Check sheet for the modelled part. Datum: model origin and axes. Units: mm. A direction names the side the tool comes from. Round coordinates to 2 decimals unless told otherwise and drop trailing zeros. Order: outer loops, then holes, each group sorted by start corner. A loop starts at its lowest first (then second) coordinate and runs counter-clockwise, first axis right, second up. Notation, with made-up numbers: (-13, 34.5) -> (29, 34.5) arc R32 cw to (29, 73.5) -> close; hole circle Ø1 at (48, 55.25). An arc over 180 degrees is marked (long way). Answer in a Markdown table with one row per item. Add a question column.
1. Material ranges on L1, parallel to Y at x = 5.25, z = 0; L2, parallel to Z at x = -0.25, y = 30.5; L3, parallel to Z at x = -4.5, y = 17.5, recorded low to high. Write a range as from..to.
2. Draft check along Z on faces 6 (the cylindrical face through (-3.51, 7.67, 4.23)), 7 (the cylindrical face through (2.6, 28.5, -0.3)), 8 (the cylindrical face through (4.904, 36.575, 0.129)). Enter one of: +Z half, -Z half, draft (parallel to the pull), parting line (faces both ways), or undercut.
3. Sectioned sample at A-A, the plane x = -3.25. Count the separate pieces of the cut face and the enclosed holes in it, then the cut area to 3 significant figures.
4. Sectioned sample at C-C, the plane z = 0. Record the boundary of the cut face in (x, y).
5. Sectioned sample at B-B, the plane z = 7.75. Record the boundary of the cut face in (x, y).
6. Depth check by flat-ended pin: P1, Ø3.5, axis at x = 2.48, y = 30.7, coming from the -Z side; P2, Ø5, axis at x = -2, y = 23.5, coming from the +Z side; P3, Ø0.6, axis at x = 3.5, y = 8, coming from the -Z side. Enter the tip coordinate at first touch or a pass-through.
7. Access from +Z, -Z, +X, -X, +Y, -Y to the whole of each face (thin tool, end or side, straight path). Record for faces 1 (the flat face through (4, 8, 5.334)), 2 (the flat face through (4, 8, -5.334)), 3 (the flat face through (-4, 17.653, 7)), 4 (the flat face through (0, 27, -5.88)), 5 (the cylindrical face through (-3.509, 7.669, -3.986)).
```python
from build123d import *

# Parameters (mm, degrees)
SKETCH1_R           = 1.905
SKETCH1_R_2         = 2.2178391
BOSS_EXTRUDE1_DEPTH = 7.76605
SKETCH2_W           = 9.0297
SKETCH2_H           = 6.858
CUT_EXTRUDE1_DEPTH  = 7.76605
CUT_EXTRUDE2_DEPTH  = 9.0297
SKETCH5_R           = 1.5875
CUT_EXTRUDE3_DEPTH  = 12.7
FILLET2_R           = 1.27
SKETCH6_W           = 4.445
SKETCH6_H           = 8.89
CUT_EXTRUDE4_DEPTH  = 8.636
SKETCH6_4_W         = 1.04775
SKETCH6_4_H         = 1.905
BOSS_EXTRUDE2_DEPTH = 15.5321
SKETCH7_R           = 2.661534018
CUT_EXTRUDE5_DEPTH  = 12.7
CUT_EXTRUDE6_DEPTH  = 8.636
CUT_EXTRUDE7_DEPTH  = 0.635
CUT_EXTRUDE8_DEPTH  = 0.635
SKETCH11_R          = 1.27
CUT_EXTRUDE9_DEPTH  = 12.7


with BuildPart() as part:
    # Sketch1 → Boss-Extrude1 (new, symmetric)
    with BuildSketch(Plane(origin=(0, 0, 0), x_dir=(0, 0, -1), z_dir=(1, 0, 0))):
        with BuildLine():
            Line((-9.779, 8.763), (-9.779, 21.463))
            Line((-9.779, 21.463), (-5.8801, 21.971))
            Line((-5.8801, 21.971), (-5.8801, 30.6959))
            ThreePointArc((-5.8801, 30.6959), (0, 36.576), (5.8801, 30.6959))
            Line((5.8801, 30.6959), (5.8801, 21.971))
            Line((5.8801, 21.971), (9.779, 21.463))
            Line((9.779, 21.463), (9.779, 8.763))
            Line((9.779, 8.763), (4.28625, 8.763))
            Line((4.28625, 8.763), (4.28625, 4.28625))
            ThreePointArc((4.28625, 4.28625), (0, 0), (-4.28625, 4.28625))
            Line((-4.28625, 4.28625), (-4.28625, 8.763))
            Line((-4.28625, 8.763), (-9.779, 8.763))
        make_face()
        with Locations(Location((0, 6.62305, 0), (0, 0, 180))):
            Circle(SKETCH1_R, mode=Mode.SUBTRACT)
        with Locations(Location((0, 30.6959, 0), (0, 0, 180))):
            Circle(SKETCH1_R_2, mode=Mode.SUBTRACT)
    extrude(amount=BOSS_EXTRUDE1_DEPTH, both=True)

    # Sketch2 → Cut-Extrude1 (cut, symmetric)
    with BuildSketch(Plane.XY):
        Polygon((3.883025, 36.576), (-7.76605, 26.33345), (-11.065137459, 26.33345), (-11.065137459, 37.341338298), align=None)
        with Locations((-3.2512, 3.429)):
            Rectangle(SKETCH2_W, SKETCH2_H)
    extrude(amount=CUT_EXTRUDE1_DEPTH, both=True, mode=Mode.SUBTRACT)

    # Sketch3 → Cut-Extrude2 (cut)
    with BuildSketch(Plane.ZY.offset(7.76605)):
        with BuildLine():
            Line((-3.65125, 6.858), (-3.65125, 3.968410348))
            Line((-3.65125, 3.968410348), (3.65125, 3.968410348))
            Line((3.65125, 3.968410348), (3.65125, 6.858))
            ThreePointArc((3.65125, 6.858), (0, 10.058441778), (-3.65125, 6.858))
        make_face()
    extrude(amount=-CUT_EXTRUDE2_DEPTH, mode=Mode.SUBTRACT)

    # Sketch5 → Cut-Extrude3 (cut, symmetric)
    with BuildSketch(Plane(origin=(0, 0, 0), x_dir=(0, 0, -1), z_dir=(1, 0, 0))):
        with Locations((-7.3025, 20.066)):
            Circle(SKETCH5_R)
        with Locations((7.3025, 20.066)):
            Circle(SKETCH5_R)
    extrude(amount=CUT_EXTRUDE3_DEPTH, both=True, mode=Mode.SUBTRACT)

    # Fillet2
    fillet2_edges = [part.edges().sort_by_distance(p)[0] for p in [
        (0, 21.971, 5.8801),
        (0, 21.971, -5.8801),
    ]]
    fillet(fillet2_edges, radius=FILLET2_R)

    # Sketch6 → Cut-Extrude4 (cut)
    with BuildSketch(Plane.ZY.offset(7.76605)):
        with Locations((-7.5565, 13.208)):
            Rectangle(SKETCH6_W, SKETCH6_H)
        with Locations((7.5565, 13.208)):
            Rectangle(SKETCH6_W, SKETCH6_H)
    extrude(amount=-CUT_EXTRUDE4_DEPTH, mode=Mode.SUBTRACT)

    # Sketch6_4 → Boss-Extrude2 (add)
    with BuildSketch(Plane.ZY.offset(7.76605)):
        with Locations((4.810125, 7.8105)):
            Rectangle(SKETCH6_4_W, SKETCH6_4_H)
        with Locations((-4.810125, 7.8105)):
            Rectangle(SKETCH6_4_W, SKETCH6_4_H)
    extrude(amount=-BOSS_EXTRUDE2_DEPTH)

    # Sketch7 → Cut-Extrude5 (cut, symmetric)
    with BuildSketch(Plane.XY):
        with Locations((-4.582517629, 12.953080778)):
            Circle(SKETCH7_R)
    extrude(amount=CUT_EXTRUDE5_DEPTH, both=True, mode=Mode.SUBTRACT)

    # Sketch8 → Cut-Extrude6 (cut)
    with BuildSketch(Plane.ZY.offset(7.76605)):
        with BuildLine():
            Line((5.334, 6.858), (5.334, 16.484599764))
            Line((5.334, 16.484599764), (4.35251984, 16.484599764))
            Line((4.35251984, 16.484599764), (4.351681885, 8.533646344))
            ThreePointArc((4.351681885, 8.533646344), (4.229677597, 7.662350207), (3.873218976, 6.858))
            Line((3.873218976, 6.858), (4.286179008, 6.858))
            Line((4.286179008, 6.858), (5.334, 6.858))
        make_face()
        with BuildLine():
            Line((-4.10568025, 16.484599736), (-5.334, 16.484599736))
            Line((-5.334, 16.484599736), (-5.334, 6.858))
            Line((-5.334, 6.858), (-3.65125, 6.858))
            ThreePointArc((-3.65125, 6.858), (-3.649079576, 6.874147348), (-3.646837743, 6.890284937))
            ThreePointArc((-3.646837743, 6.890284937), (-3.988818984, 7.680928893), (-4.10568025, 8.534399736))
            Line((-4.10568025, 8.534399736), (-4.10568025, 16.484599736))
        make_face()
    extrude(amount=-CUT_EXTRUDE6_DEPTH, mode=Mode.SUBTRACT)

    # Sketch9 → Cut-Extrude7 (cut)
    with BuildSketch(Plane.XY.offset(9.779)):
        Polygon((-2.899226122, 16.483160278), (0.86995, 16.483160278), (0.86995, 17.653), (-7.76605, 17.653), (-7.76605, 21.463), (0.86995, 21.463), (0.86995, 24.857620894), (-13.663084866, 24.857620894), (-13.663084866, 16.483160278), (-7.00405, 16.483160278), (-3.833922711, 16.483160278), align=None)
        Polygon((-7.76605, 17.653), (0.86995, 17.653), (0.86995, 20.039153951), (0.86995, 21.463), (-7.76605, 21.463), align=None)
    extrude(amount=-CUT_EXTRUDE7_DEPTH, mode=Mode.SUBTRACT)

    # Sketch10 → Cut-Extrude8 (cut)
    with BuildSketch(Plane(origin=(0, 0, -9.779), x_dir=(-1, 0, 0), z_dir=(0, 0, -1))):
        Polygon((3.833922711, 16.483160278), (7.00405, 16.483160278), (13.663084866, 16.483160278), (13.663084866, 24.857620894), (-0.86995, 24.857620894), (-0.86995, 20.039153951), (-0.86995, 17.653), (-0.86995, 16.483160278), (2.899226122, 16.483160278), align=None)
    extrude(amount=-CUT_EXTRUDE8_DEPTH, mode=Mode.SUBTRACT)

    # Sketch11 → Cut-Extrude9 (cut, symmetric)
    with BuildSketch(Plane.XY):
        with Locations((2.480754657, 30.6959)):
            Circle(SKETCH11_R)
    extrude(amount=CUT_EXTRUDE9_DEPTH, both=True, mode=Mode.SUBTRACT)


solid = part.part
```
Answer key:
| question | item | result |
|---|---|---|
| 1 | L1 | y = 0..4.72, 8.53..28.48, 32.91..36.58 |
| 1 | L2 | z = -5.88..-2.21, 2.21..5.88 |
| 1 | L3 | z = -5.33..5.33 |
| 2 | face 6 | +Z half |
| 2 | face 7 | undercut |
| 2 | face 8 | parting line |
| 3 | separate pieces | 2 |
| 3 | enclosed holes | 2 |
| 3 | area | 191 mm² |
| 4 | outline | (-7.77, 10.06) -> (1.26, 10.06) -> (1.26, 8.53) -> (7.77, 8.53) -> (7.77, 28.48) -> (-5.33, 28.48) -> (-7.77, 26.33) -> close; (-0.28, 32.91) -> (7.77, 32.91) -> (7.77, 36.58) -> (3.88, 36.58) -> close; (1.26, 0) -> (7.77, 0) -> (7.77, 4.72) -> (1.26, 4.72) -> close; hole circle Ø5.32 at (-4.58, 12.95) |
| 5 | outline | (-7.77, 17.65) -> (0.87, 17.65) -> (0.87, 8.76) -> (7.77, 8.76) -> (7.77, 18.54) -> (-7.77, 18.54) -> close; (-7.77, 21.59) -> (7.77, 21.59) -> (7.77, 21.73) -> (-7.77, 21.73) -> close |
| 6 | P1 | stops at z = -5.88 |
| 6 | P2 | stops at z = 9.14 |
| 6 | P3 | stops at z = -5.33 |
| 7 | face 1 | +Z, +X, -X, -Y |
| 7 | face 2 | -Z, +X, -X, -Y |
| 7 | face 3 | +Z, -X, -Y |
| 7 | face 4 | -Z, +X, -X, +Y |
| 7 | face 5 | -Z, -X, -Y |
